Geometry: final body of the model. Coordinates: model frame, mm. A direction names the side the tool comes from. Coordinates: 2 decimals unless noted, no trailing zeros. Write each loop counter-clockwise with the first axis right and the second up, starting at its lowest first coordinate (ties: lowest second). Pieces come first, ordered by that corner, then holes.
from build123d import *

# Parameters (mm, degrees)
SKETCH1_W               = 138
SKETCH1_H               = 40
SKETCH1_W_2             = 41
SKETCH1_H_2             = 21
BOSS_EXTRUDE1_DEPTH     = 12
FILLET1_RADIUS          = 20
FILLET1_LENGTH          = 12
FILLET2_RADIUS          = 20
FILLET2_LENGTH          = 12
BOSS_EXTRUDE3_START     = 7
BOSS_EXTRUDE3_DEPTH     = 7
BOSS_EXTRUDE4_START     = 7
BOSS_EXTRUDE4_DEPTH     = 7
CUT_EXTRUDE1_DEPTH      = 75.310160813
CUT_EXTRUDE1_DEPTH_BACK = 75.310160813
CUT_EXTRUDE2_DEPTH      = 2.5
SKETCH9_W               = 41
SKETCH9_H               = 21
CUT_EXTRUDE3_DEPTH      = 2.5
SKETCH10_W              = 41
SKETCH10_H              = 21
SKETCH10_R              = 7.5
BOSS_EXTRUDE5_DEPTH     = 2
SKETCH11_W              = 41
SKETCH11_H              = 21
SKETCH11_R              = 7.5
BOSS_EXTRUDE6_DEPTH     = 2
SKETCH12_W              = 4
SKETCH12_H              = 1
CUT_EXTRUDE4_DEPTH      = 2
SKETCH13_W              = 3
SKETCH13_H              = 1
CUT_EXTRUDE5_DEPTH      = 2
FILLET4_R               = 2
FILLET5_R               = 2
FILLET6_R               = 1
SKETCH14_R              = 1.4
CUT_EXTRUDE6_DEPTH      = 74.71058283
SKETCH15_R              = 1.4
CUT_EXTRUDE7_DEPTH      = 74.71058283


with BuildPart() as part:
    # Sketch1 → Boss-Extrude1 (new body)
    with BuildSketch(Plane.XY):
        Rectangle(SKETCH1_W, SKETCH1_H)
        with Locations((-33.5, 0)):
            Rectangle(SKETCH1_W_2, SKETCH1_H_2, mode=Mode.SUBTRACT)
        with Locations((33.5, 0)):
            Rectangle(SKETCH1_W_2, SKETCH1_H_2, mode=Mode.SUBTRACT)
    extrude(amount=BOSS_EXTRUDE1_DEPTH)

    # Fillet1: full round fillet: the end face becomes a half cylinder, R = half its width
    fillet1_face = Plane((-69, 0, 6), x_dir=(0, 0, 1), z_dir=(-1, 0, 0))  # on the end face: x along it, z out of the body
    fillet1_slab = fillet1_face.offset(-FILLET1_RADIUS / 2) * Box(FILLET1_LENGTH, 2 * FILLET1_RADIUS, FILLET1_RADIUS, mode=Mode.PRIVATE)  # the body's end, R deep
    fillet1_round = Plane((-49, 0, 6), x_dir=(-1, 0, 0), z_dir=(0, 0, 1)) * Cylinder(FILLET1_RADIUS, FILLET1_LENGTH, mode=Mode.PRIVATE)  # its axis R under the face
    add(fillet1_slab - fillet1_round, mode=Mode.SUBTRACT)

    # Fillet2: full round fillet: the end face becomes a half cylinder, R = half its width
    fillet2_face = Plane((69, 0, 6), x_dir=(0, 0, -1), z_dir=(1, 0, 0))  # on the end face: x along it, z out of the body
    fillet2_slab = fillet2_face.offset(-FILLET2_RADIUS / 2) * Box(FILLET2_LENGTH, 2 * FILLET2_RADIUS, FILLET2_RADIUS, mode=Mode.PRIVATE)  # the body's end, R deep
    fillet2_round = Plane((49, 0, 6), x_dir=(1, 0, 0), z_dir=(0, 0, -1)) * Cylinder(FILLET2_RADIUS, FILLET2_LENGTH, mode=Mode.PRIVATE)  # its axis R under the face
    add(fillet2_slab - fillet2_round, mode=Mode.SUBTRACT)

    # Sketch3 → Boss-Extrude3 (add)
    with BuildSketch(Plane.XY.offset(12).offset(BOSS_EXTRUDE3_START)):
        with BuildLine():
            Line((-49, -20), (-2.5, -20))
            Line((-2.5, -20), (2.5, -20))
            Line((2.5, -20), (2.5, 20))
            Line((2.5, 20), (-2.5, 20))
            Line((-2.5, 20), (-49, 20))
            ThreePointArc((-49, 20), (-69, 0), (-49, -20))
        make_face()
        with BuildLine():
            Line((-2.5, 17), (-2.5, -17))
            Line((-2.5, -17), (-49, -17))
            ThreePointArc((-49, -17), (-66, 0), (-49, 17))
            Line((-49, 17), (-2.5, 17))
        make_face(mode=Mode.SUBTRACT)
    extrude(amount=-BOSS_EXTRUDE3_DEPTH)

    # Sketch5 → Boss-Extrude4 (add)
    with BuildSketch(Plane(origin=(0, 0, 0), x_dir=(-1, 0, 0), z_dir=(0, 0, -1)).offset(BOSS_EXTRUDE4_START)):
        with BuildLine():
            Line((-49, -20), (-2.5, -20))
            Line((-2.5, -20), (2.5, -20))
            Line((2.5, -20), (2.5, 20))
            Line((2.5, 20), (-2.5, 20))
            Line((-2.5, 20), (-49, 20))
            ThreePointArc((-49, 20), (-69, 0), (-49, -20))
        make_face()
        with BuildLine():
            Line((-2.5, 17), (-2.5, -17))
            Line((-2.5, -17), (-49, -17))
            ThreePointArc((-49, -17), (-66, 0), (-49, 17))
            Line((-49, 17), (-2.5, 17))
        make_face(mode=Mode.SUBTRACT)
    extrude(amount=-BOSS_EXTRUDE4_DEPTH)

    # Sketch6 → Cut-Extrude1 (cut, two sides: drawn at the far end of the back side and taken through both)
    with BuildSketch(Plane(origin=(0, 0, 0), x_dir=(1, 0, 0), z_dir=(0, 1, 0)).offset(-CUT_EXTRUDE1_DEPTH_BACK)):
        with BuildLine():
            Line((-69, -19), (-29, -19))
            add(Edge.make_bspline(
                [(-69, -14), (-48.966763925, -16.237598457), (-29, -19)],
                knots=[0, 0, 0, 1, 1, 1], degree=2))
            Line((-69, -14), (-69, -19))
        make_face()
        with BuildLine():
            Line((69, 7), (29, 7))
            add(Edge.make_bspline(
                [(69, 2), (48.966763925, 4.237598457), (29, 7)],
                knots=[0, 0, 0, 1, 1, 1], degree=2))
            Line((69, 2), (69, 7))
        make_face()
    extrude(amount=CUT_EXTRUDE1_DEPTH + CUT_EXTRUDE1_DEPTH_BACK, mode=Mode.SUBTRACT)

    # Sketch8 → Cut-Extrude2 (cut)
    with BuildSketch(Plane.XY.offset(12)):
        with BuildLine():
            Line((-49, -17), (-2.5, -17))
            Line((-2.5, -17), (-2.5, 17))
            Line((-2.5, 17), (-29, 17))
            Line((-29, 17), (-49, 17))
            ThreePointArc((-49, 17), (-66, 0), (-49, -17))
        make_face()
    extrude(amount=-CUT_EXTRUDE2_DEPTH, mode=Mode.SUBTRACT)

    # Sketch9 → Cut-Extrude3 (cut)
    with BuildSketch(Plane(origin=(0, 0, 0), x_dir=(-1, 0, 0), z_dir=(0, 0, -1))):
        with BuildLine():
            ThreePointArc((-49, 17), (-66, 0), (-49, -17))
            Line((-49, -17), (-2.5, -17))
            Line((-2.5, -17), (-2.5, 17))
            Line((-2.5, 17), (-29, 17))
            Line((-29, 17), (-49, 17))
        make_face()
        with Locations((-33.5, 0)):
            Rectangle(SKETCH9_W, SKETCH9_H, mode=Mode.SUBTRACT)
    extrude(amount=-CUT_EXTRUDE3_DEPTH, mode=Mode.SUBTRACT)

    # Sketch10 → Boss-Extrude5 (add)
    with BuildSketch(Plane.XY.offset(12)):
        with Locations((33.5, 0)):
            Rectangle(SKETCH10_W, SKETCH10_H)
        with Locations((44.09, 0)):
            Circle(SKETCH10_R, mode=Mode.SUBTRACT)
    extrude(amount=-BOSS_EXTRUDE5_DEPTH)

    # Sketch11 → Boss-Extrude6 (add)
    with BuildSketch(Plane(origin=(0, 0, 0), x_dir=(-1, 0, 0), z_dir=(0, 0, -1))):
        with Locations((33.5, 0)):
            Rectangle(SKETCH11_W, SKETCH11_H)
        with Locations((44.09, 0)):
            Circle(SKETCH11_R, mode=Mode.SUBTRACT)
    extrude(amount=-BOSS_EXTRUDE6_DEPTH)

    # Sketch12 → Cut-Extrude4 (cut)
    with BuildSketch(Plane.XY.offset(9.5)):
        with Locations((-56, 0)):
            Rectangle(SKETCH12_W, SKETCH12_H)
        with Locations((-11, 0)):
            Rectangle(SKETCH12_W, SKETCH12_H)
    extrude(amount=-CUT_EXTRUDE4_DEPTH, mode=Mode.SUBTRACT)

    # Sketch13 → Cut-Extrude5 (cut)
    with BuildSketch(Plane(origin=(0, 0, 2.5), x_dir=(-1, 0, 0), z_dir=(0, 0, -1))):
        with Locations((-55.5, 0)):
            Rectangle(SKETCH13_W, SKETCH13_H)
        with Locations((-11.5, 0)):
            Rectangle(SKETCH13_W, SKETCH13_H)
    extrude(amount=-CUT_EXTRUDE5_DEPTH, mode=Mode.SUBTRACT)

    # Fillet4
    fillet4_edges = [part.edges().sort_by_distance(p)[0] for p in [
        (2.5, 0, 12),
    ]]
    fillet(fillet4_edges, radius=FILLET4_R)

    # Fillet5
    fillet5_edges = [part.edges().sort_by_distance(p)[0] for p in [
        (-2.5, 0, 0),
    ]]
    fillet(fillet5_edges, radius=FILLET5_R)

    # Fillet6
    fillet6_edges = [part.edges().sort_by_distance(p)[0] for p in [
        (2.5, 0, 19),
        (-2.5, 0, -7),
    ]]
    fillet(fillet6_edges, radius=FILLET6_R)

    # Sketch14 → Cut-Extrude6 (cut, through all)
    with BuildSketch(Plane(origin=(0, 0, 2.5), x_dir=(-1, 0, 0), z_dir=(0, 0, -1))):
        with Locations((-57.5, 5)):
            Circle(SKETCH14_R)
        with Locations((-57.5, -5)):
            Circle(SKETCH14_R)
        with Locations((-9.5, 5)):
            Circle(SKETCH14_R)
        with Locations((-9.5, -5)):
            Circle(SKETCH14_R)
    extrude(amount=-CUT_EXTRUDE6_DEPTH, mode=Mode.SUBTRACT)

    # Sketch15 → Cut-Extrude7 (cut, through all)
    with BuildSketch(Plane.XY.offset(9.5)):
        with Locations((-57.5, 5)):
            Circle(SKETCH15_R)
        with Locations((-57.5, -5)):
            Circle(SKETCH15_R)
        with Locations((-9.5, -5)):
            Circle(SKETCH15_R)
        with Locations((-9.5, 5)):
            Circle(SKETCH15_R)
    extrude(amount=-CUT_EXTRUDE7_DEPTH, mode=Mode.SUBTRACT)


solid = part.part
Item 1: Set-up query: faces 1 (the flat face through (25, -17, -2)), 2 (the cylindrical face through (56.165, 5.421, 7.184)), 3 (the flat face through (-54, 0, 6)), 4 (the flat face through (-2.5, 0, -4)), 5 (the flat face through (2.5, 0, 16)). Return all of +Z, -Z, +X, -X, +Y, -Y with unobstructed straight access to the full face (end or side cutting, diameter ignored); none if empty.
Derived:
face 1: -Z
face 2: +Z, -Z
face 3: +Z
face 4: -Z, -X, +Y, -Y
face 5: +Z, +X, +Y, -Y
Item 2: Material intervals for probe 1 along Y at (x, z) = (9.5, 7); probe 2 along X at (y, z) = (-8.5, 2.75); probe 3 along Y at (x, z) = (24, 0.75), sorted ascending.
Derived:
probe 1: y = -20 to -6.4, -3.6 to 3.6, 6.4 to 20
probe 2: x = -67.1 to -54, -13 to 13, 54 to 67.1
probe 3: y = -20 to -17, 17 to 20
Item 3: Section A-A, the plane z = 5.75. State how many separate pieces and enclosed holes the cut face has, plus the area to 3 significant figures.
Derived:
separate pieces: 1
enclosed holes: 10
area: 3,410 mm2
Item 4: Section B-B, the plane x = -15. Output: boundary loops of the cut face in (y, z).
Derived:
outline: (-20, 0) - (20, 0) - (20, 19) - (17, 19) - (17, 9.5) - (10.5, 9.5) - (10.5, 2) - (-10.5, 2) - (-10.5, 9.5) - (-17, 9.5) - (-17, 19) - (-20, 19) - close
Item 5: Pull-direction query (Y, two-part tool) for faces 6 (the flat face through (-29, 0, 2)), 7 (the cylindrical face through (-69, 0, 8)), 8 (the flat face through (36, 0, 12)); classes: released by +Y, released by -Y, zero draft, split by the parting line, or undercut.
Derived:
face 6: undercut
face 7: split by the parting line
face 8: zero draft
Item 6: Pin query (flat end, axial travel): pin 1 (1 mm diameter, centred on x = 50.5, y = 16, fed in from +Z); pin 2 (5 mm diameter, centred on y = 4.5, z = 14, fed in from +X); pin 3 (3 mm diameter, centred on x = 57.5, y = 5, fed in from -Z); pin 4 (6 mm diameter, centred on y = 1.5, z = 5, fed in from +X). Return the tip coordinate at first contact, or that it passes through.
Derived:
pin 1: stops at z = 12
pin 2: stops at x = 68.77
pin 3: stops at z = 2.5
pin 4: stops at x = 69
